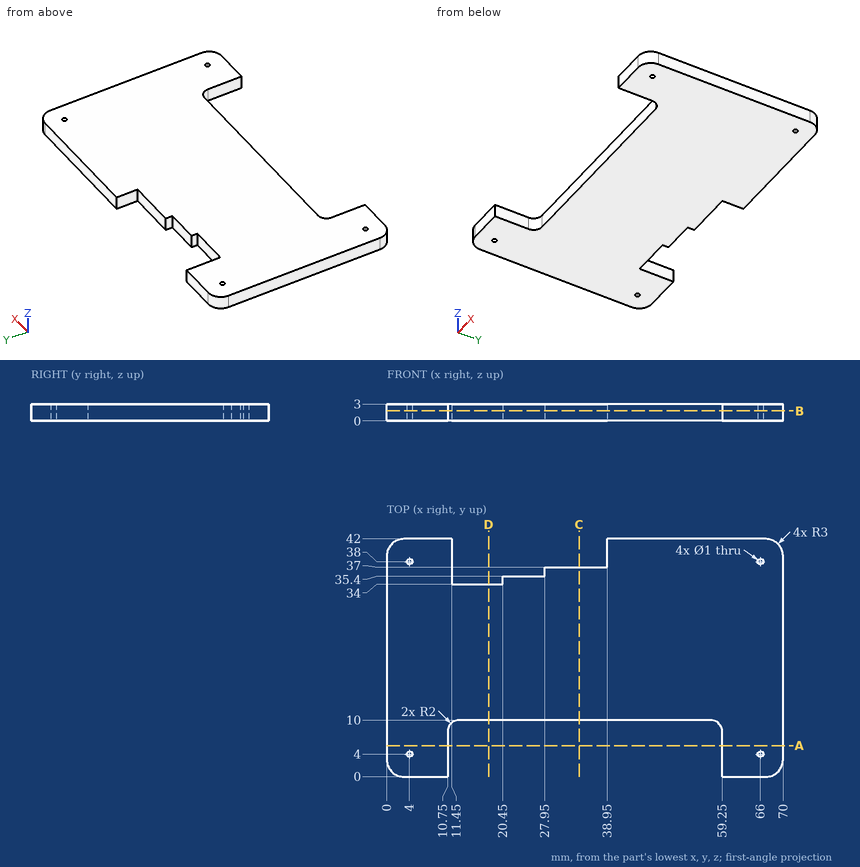
Check sheet for the drawn part. Datum: minimum x, y, z corner. Units: mm. Round coordinates to 2 decimals unless told otherwise and drop trailing zeros. Write each loop counter-clockwise with the first axis right and the second up, starting at its lowest first coordinate (ties: lowest second). Pieces come first, ordered by that corner, then holes. Notation, with made-up numbers: (50, 64) - (56, 64) arc R28 ccw to (56, 84) - close; hole circle Ø4 at (20, 46). An arc over 180 degrees is marked (long way). Write each question's results on one line, items separated by ' | '.
(1) Thickness scan on probe 1 along Y at (x, z) = (4, 2.05); probe 2 along X at (y, z) = (38, 1.3); probe 3 along X at (y, z) = (7.5, 2.25). Record the ranges inside material, lowest first. Write a range as from..to.
Computed:
probe 1: y = 0..3.5, 4.5..37.5, 38.5..42 | probe 2: x = 0..3.5, 4.5..11.45, 38.95..65.5, 66.5..70 | probe 3: x = 0..10.75, 59.25..70
(2) Depth check by flat-ended pin: pin 1 Ø1.5 at (x, z) = (22.5, 2) entering from +Y; pin 2 Ø0.9 at (x, z) = (16.5, 1.5) entering from +Y; pin 3 Ø0.9 at (y, z) = (40.5, 1.5) entering from -X. Enter the tip coordinate at first touch or a pass-through.
Computed:
pin 1: stops at y = 35.4 | pin 2: stops at y = 34 | pin 3: stops at x = 0.19
(3) Sectioned sample at B-B, the plane z = 1.8. Enter the section's corners in (x, y).
Computed:
outline: (0, 3) arc R3 ccw to (3, 0) - (10.75, 0) - (10.75, 8) arc R2 cw to (12.75, 10) - (57.25, 10) arc R2 cw to (59.25, 8) - (59.25, 0) - (67, 0) arc R3 ccw to (70, 3) - (70, 39) arc R3 ccw to (67, 42) - (38.95, 42) - (38.95, 37) - (27.95, 37) - (27.95, 35.4) - (20.45, 35.4) - (20.45, 34) - (11.45, 34) - (11.45, 42) - (3, 42) arc R3 ccw to (0, 39) - close; hole circle Ø1 at (4, 4); hole circle Ø1 at (4, 38); hole circle Ø1 at (66, 4); hole circle Ø1 at (66, 38)
(4) Sectioned sample at D-D, the plane x = 18. Enter the section's corners in (y, z).
Computed:
outline: (10, 0) - (34, 0) - (34, 3) - (10, 3) - close
(5) Sectioned sample at A-A, the plane y = 5.5. Enter the section's corners in (x, z).
Computed:
outline: (0, 0) - (10.75, 0) - (10.75, 3) - (0, 3) - close; (59.25, 0) - (70, 0) - (70, 3) - (59.25, 3) - close
(6) Sectioned sample at C-C, the plane x = 34. Enter the section's corners in (y, z).
Computed:
outline: (10, 0) - (37, 0) - (37, 3) - (10, 3) - close
